Design review of the part built by this model. Coordinates are the model's own, in mm. Face numbers are marked on the shaded views. A direction names the side the tool comes from. Coordinates: 2 decimals unless noted, no trailing zeros. Loops run counter-clockwise (first coordinate to the right, second up) from the corner with the lowest first, then second, coordinate; pieces in that order, holes last. Notation, with made-up numbers: (51, 7) -> (70, 7) arc R24 cw to (70, 27) -> close; hole circle Ø6 at (45.25, 67.25). An arc over 180 degrees is marked (long way). Use CSV: the item, a comma, the result in double quotes.
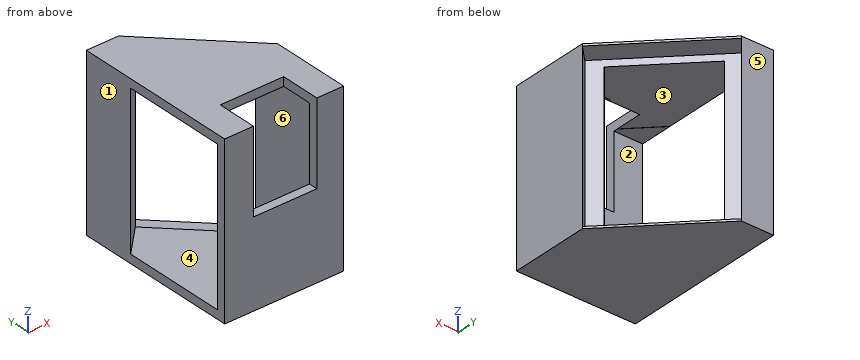
```python
from build123d import *

# Parameters (mm, degrees)
SKETCH1_W               = 150
SKETCH1_H               = 150
BOSS_EXTRUDE2_DEPTH     = 152
CHAMFER1_SIZE           = 78.48885271
SKETCH4_W               = 148.25
SKETCH4_H               = 111
CUT_EXTRUDE5_DEPTH      = 19
SKETCH5_W               = 136.25
SKETCH5_H               = 84
CUT_EXTRUDE6_DEPTH      = 81
CUT_EXTRUDE7_DEPTH      = 20
CUT_EXTRUDE7_DEPTH_BACK = 153
SKETCH6_W               = 42.53672634
SKETCH6_H               = 150
SKETCH7_W               = 136.153133976
SKETCH7_H               = 29.553064713
CUT_EXTRUDE8_DEPTH      = 84
SKETCH8_W               = 136.25
SKETCH8_H               = 30.070372941
CUT_EXTRUDE9_DEPTH      = 30
SKETCH9_W               = 57.3
SKETCH9_H               = 36
CUT_EXTRUDE10_DEPTH     = 74.6


with BuildPart() as part:
    # Sketch1 → Boss-Extrude2 (new body)
    with BuildSketch(Plane.XY):
        with Locations((75, 75)):
            Rectangle(SKETCH1_W, SKETCH1_H)
    extrude(amount=BOSS_EXTRUDE2_DEPTH)

    # Chamfer1
    chamfer1_edges = [part.edges().sort_by_distance(p)[0] for p in [
        (150, 150, 76),
    ]]
    chamfer(chamfer1_edges, length=CHAMFER1_SIZE)

    # Sketch4 → Cut-Extrude5 (cut)
    with BuildSketch(Plane(origin=(110.755573645, 110.755573645, 0), x_dir=(0, 0, -1), z_dir=(0.7071067811865489, 0.7071067811865461, 0))):
        with Locations((-76, 0.001948307)):
            Rectangle(SKETCH4_W, SKETCH4_H)
    extrude(amount=-CUT_EXTRUDE5_DEPTH, mode=Mode.SUBTRACT)

    # Sketch5 → Cut-Extrude6 (cut)
    with BuildSketch(Plane(origin=(97.320544802, 97.320544802, 0), x_dir=(0, 0, -1), z_dir=(0.707106781186549, 0.707106781186546, 0))):
        with Locations((-76, 0.001948307)):
            Rectangle(SKETCH5_W, SKETCH5_H)
    extrude(amount=-CUT_EXTRUDE6_DEPTH, mode=Mode.SUBTRACT)

    # Sketch6 → Cut-Extrude7 (cut, two sides: drawn at the far end of the back side and taken through both)
    with BuildSketch(Plane.XY.offset(152).offset(-CUT_EXTRUDE7_DEPTH_BACK)):
        with Locations((21.26836317, 75)):
            Rectangle(SKETCH6_W, SKETCH6_H)
    extrude(amount=CUT_EXTRUDE7_DEPTH + CUT_EXTRUDE7_DEPTH_BACK, mode=Mode.SUBTRACT)

    # Sketch7 → Cut-Extrude8 (cut)
    with BuildSketch(Plane.ZY.offset(-42.53672634)):
        with Locations((75.951566988, 22.776532357)):
            Rectangle(SKETCH7_W, SKETCH7_H)
    extrude(amount=-CUT_EXTRUDE8_DEPTH, mode=Mode.SUBTRACT)

    # Sketch8 → Cut-Extrude9 (cut)
    with BuildSketch(Plane.ZY.offset(-126.53672634)):
        with Locations((76, 52.588251184)):
            Rectangle(SKETCH8_W, SKETCH8_H)
    extrude(amount=CUT_EXTRUDE9_DEPTH, mode=Mode.SUBTRACT)

    # Sketch9 → Cut-Extrude10 (cut)
    with BuildSketch(Plane.XY.offset(152)):
        with Locations((97.18672634, 18)):
            Rectangle(SKETCH9_W, SKETCH9_H)
    extrude(amount=-CUT_EXTRUDE10_DEPTH, mode=Mode.SUBTRACT)


solid = part.part
```
Item 1: Draft analysis for pull direction Y (two halves, no side actions). For the marked faces 4, 5 and 6, state which applies: pulls with the +Y half, pulls with the -Y half, needs draft (parallel to the pull), parting line crosses it, or undercut.
Checked values:
face 4,"undercut"
face 5,"pulls with the +Y half"
face 6,"needs draft"
Item 2: Add section D-D (y = 63.5). Give the boundary of the cut face in (x, z) (3 decimals).
Checked values:
outline,"(42.537, 0) -> (150, 0) -> (150, 152) -> (42.537, 152) -> (42.537, 144.125) -> (126.537, 144.125) -> (126.537, 7.875) -> (42.537, 7.875) -> close; hole (131.141, 1.875) -> (141.986, 1.875) -> (141.986, 150.125) -> (131.141, 150.125) -> close"
Item 3: Add section B-B (x = 112.5). Give the boundary of the cut face in (y, z) (3 decimals).
Checked values:
outline,"(0, 0) -> (109.011, 0) -> (109.011, 1.875) -> (82.141, 1.875) -> (82.141, 7.875) -> (8, 7.875) -> (8, 77.4) -> (0, 77.4) -> close; (36, 144.028) -> (37.553, 144.028) -> (37.553, 144.125) -> (82.141, 144.125) -> (82.141, 150.125) -> (109.011, 150.125) -> (109.011, 152) -> (36, 152) -> close"
Item 4: Machinability: for the marked faces 1, 2 and 3, which of the approach directions +Z, -Z, +X, -X, +Y, -Y give a long, thin tool a straight path to every point of the face, cutting with its end or side? Answer none if there is none.
Checked values:
face 1,"+Z, -Z, -X, +Y, -Y"
face 2,"-X"
face 3,"none"
Item 5: To check wall thickness, follow line 1 along Z through (x, y) = (106, 79.5) (3 decimals); line 2 along Z through (x, y) = (120.5, 86.5) (3 decimals); line 3 along X through (y, z) = (6, 102.5). State the ranges of each line that lie inside material, in increasing order.
Checked values:
line 1,"0 to 7.875, 144.125 to 152"
line 2,"0 to 1.875, 150.125 to 152"
line 3,"42.54 to 68.54, 125.84 to 150"
Item 6: Add section C-C (z = 115). State how many separate pieces and enclosed holes the cut face has, then the cut area to 3 significant figures.
Checked values:
separate pieces,"3"
enclosed holes,"0"
area,"2,520 mm^2"
Item 7: Clearance check with flat-ended pins moving along their axes: pin 1 (6 mm diameter, centred on y = 104, z = 16, fed in from +X); pin 2 (10 mm diameter, centred on x = 139, z = 134.5, fed in from +Y); pin 3 (6.5 mm diameter, centred on x = 108, y = 2.5, fed in from +Z). State where each tip first meets the part, or that it passes through.
Checked values:
pin 1,"x = 47.6"
pin 2,"y = 65.51"
pin 3,"z = 77.4"
